Geometry: final body of the model. Coordinates: model frame, mm. A direction names the side the tool comes from. Round coordinates to 2 decimals unless told otherwise and drop trailing zeros. Loops run counter-clockwise (first coordinate to the right, second up) from the corner with the lowest first, then second, coordinate; pieces in that order, holes last. Notation, with made-up numbers: (45, 51.5) - (95, 51.5) arc R34 ccw to (95, 86.5) - close; hole circle Ø11 at (62.25, -17.75). An arc over 180 degrees is marked (long way). Answer in a Markdown table with one row per item. Add a question column.
from build123d import *

# Parameters (mm, degrees)
F1_DEPTH = 12.7
F2_W     = 35.4655683041
F2_H     = 12.740496546
F3_DEPTH = 76.2
F5_DEPTH = 25.4
F7_DEPTH = 12.7


with BuildPart() as f1:
    # F0 (on Top) → F1 (new body)
    with BuildSketch(Plane.XY):
        with BuildLine():
            Line((-17.732784152, -30.9358154462), (-17.732784152, -32.9542048275))
            Line((-17.732784152, -32.9542048275), (17.732784152, -32.9542048275))
            Line((17.732784152, -32.9542048275), (17.732784152, -30.9358154462))
            ThreePointArc((17.732784152, -30.9358154462), (0, -14.1835319409), (-17.732784152, -30.9358154462))
        make_face()
        with BuildLine():
            ThreePointArc((-17.732784152, -30.9358154462), (-17.761478196, -31.9450101369), (-17.732784152, -32.9542048275))
            Line((-17.732784152, -32.9542048275), (-17.732784152, -30.9358154462))
        make_face()
        with BuildLine():
            Line((17.732784152, -32.9542048275), (-17.732784152, -32.9542048275))
            ThreePointArc((-17.732784152, -32.9542048275), (0, -49.7064883328), (17.732784152, -32.9542048275))
        make_face()
        with BuildLine():
            Line((17.732784152, -30.9358154462), (17.732784152, -32.9542048275))
            ThreePointArc((17.732784152, -32.9542048275), (17.7543032358, -32.4498114027), (17.761478196, -31.9450101369))
            ThreePointArc((17.761478196, -31.9450101369), (17.7543032358, -31.440208871), (17.732784152, -30.9358154462))
        make_face()
        with BuildLine():
            Line((-17.732784152, 32.9542048275), (-17.732784152, -30.9358154462))
            ThreePointArc((-17.732784152, -30.9358154462), (0, -14.1835319409), (17.732784152, -30.9358154462))
            Line((17.732784152, -30.9358154462), (17.732784152, 32.9542048275))
            Line((17.732784152, 32.9542048275), (-17.732784152, 32.9542048275))
        make_face()
    extrude(amount=F1_DEPTH)

    # F2 (on face) → F3 (join)
    with BuildSketch(Plane.XY.offset(12.7)):
        with Locations((0, 26.5839565545)):
            Rectangle(F2_W, F2_H)
    extrude(amount=F3_DEPTH)

    # F4 (on face) → F5 (cut)
    with BuildSketch(Plane.XZ.offset(-20.2137082815)):
        with BuildLine():
            Line((5.032784152, 88.9), (-5.032784152, 88.9))
            Line((-5.032784152, 88.9), (-5.032784152, 71.3885948062))
            ThreePointArc((-5.032784152, 71.3885948062), (0, 75.6482347117), (5.032784152, 71.3885948062))
            Line((5.032784152, 71.3885948062), (5.032784152, 88.9))
        make_face()
        with BuildLine():
            ThreePointArc((5.032784152, 71.3885948062), (0, 75.6482347117), (-5.032784152, 71.3885948062))
            Line((-5.032784152, 71.3885948062), (5.032784152, 71.3885948062))
        make_face()
        with BuildLine():
            Line((5.032784152, 71.3885948062), (-5.032784152, 71.3885948062))
            ThreePointArc((-5.032784152, 71.3885948062), (-0.4231113675, 65.4599085761), (5.1029487715, 70.5452859402))
            ThreePointArc((5.1029487715, 70.5452859402), (5.0853773641, 70.9683973077), (5.032784152, 71.3885948062))
        make_face()
    extrude(amount=-F5_DEPTH, mode=Mode.SUBTRACT)

    # F6 (on face) → F7 (cut)
    with BuildSketch(Plane.YZ.offset(17.732784152)):
        Polygon((0, 0), (32.9542048275, 0), (32.9542048275, 28.4884087741), (20.2137082815, 28.4884087741), (20.2137082815, 12.7), (0, 12.7), align=None)
    extrude(amount=-F7_DEPTH, mode=Mode.SUBTRACT)


solid = f1.part
1) Section B-B, the plane z = 67. Return the cut outline in (x, y), and give its area (3 significant figures).
2) Reachability of faces 4 (the flat face through (11, 27, 28.488)), 5 (the flat face through (0, 20.214, 50)), 6 (the flat face through (11, 0, 6)), 7 (the flat face through (-5.033, 26, 80)), 8 (the flat face through (5.033, 20, 11)) from +Z, -Z, +X, -X, +Y, -Y: full face, straight path, thin tool, end or side. Return the list, or none.
3) Pull-direction query (X, two-part tool) for faces 1 (the flat face through (0, 32.954, 44)), 2 (the flat face through (5.033, 26, 80)), 3 (the flat face through (17.733, -16, 6)); classes: pulls with the +X half, pulls with the -X half, needs draft (parallel to the pull), parting line crosses it, or undercut.
4) Material intervals for line 1 along Y through (x, z) = (-16, 35.5); line 2 along Z through (x, y) = (0, 26); line 3 along Z through (x, y) = (10, -43), sorted ascending. Write a range as from..to.
5) Section C-C, the plane y = -22. Return the cut outline in (x, z).
6) Section D-D, the plane z = 58. Return the cut outline in (x, y), and give its area (3 significant figures).
7) Contact query for flat-ended pins moving along their axis: pin 1 Ø4 at (x, y) = (12.5, 29) entering from -Z; pin 2 Ø6.5 at (y, z) = (26.5, 64.5) entering from +X; pin 3 Ø10 at (y, z) = (1, 9.5) entering from -X; pin 4 Ø6 at (x, z) = (0, 70.55) entering from +Y. Output: stop coordinate, or through.
8) Section A-A, the plane x = 0. Return the cut outline in (y, z), and give its area (3 significant figures).
Evaluation:
| question | item | result |
|---|---|---|
| 1 | outline | (-17.73, 20.21) - (-3.67, 20.21) - (-3.67, 32.95) - (-17.73, 32.95) - close; (3.67, 20.21) - (17.73, 20.21) - (17.73, 32.95) - (3.67, 32.95) - close |
| 1 | area | 358 mm² |
| 2 | face 4 | -Z, +X, +Y, -Y |
| 2 | face 5 | +Z, +X, -X, -Y |
| 2 | face 6 | +Z, -Z, +X, +Y |
| 2 | face 7 | +Z, +Y, -Y |
| 2 | face 8 | -Z, +X, +Y |
| 3 | face 1 | needs draft |
| 3 | face 2 | undercut |
| 3 | face 3 | pulls with the +X half |
| 4 | line 1 | y = 20.21..32.95 |
| 4 | line 2 | z = 0..65.44 |
| 4 | line 3 | z = 0..12.7 |
| 5 | outline | (-17.73, 0) - (17.73, 0) - (17.73, 12.7) - (-17.73, 12.7) - close |
| 6 | outline | (-17.73, 20.21) - (17.73, 20.21) - (17.73, 32.95) - (-17.73, 32.95) - close |
| 6 | area | 452 mm² |
| 7 | pin 1 | stops at z = 28.49 |
| 7 | pin 2 | stops at x = 17.73 |
| 7 | pin 3 | stops at x = -17.73 |
| 7 | pin 4 | passes through |
| 8 | outline | (-49.71, 0) - (32.95, 0) - (32.95, 65.44) - (20.21, 65.44) - (20.21, 12.7) - (-49.71, 12.7) - close |
| 8 | area | 1,720 mm² |
